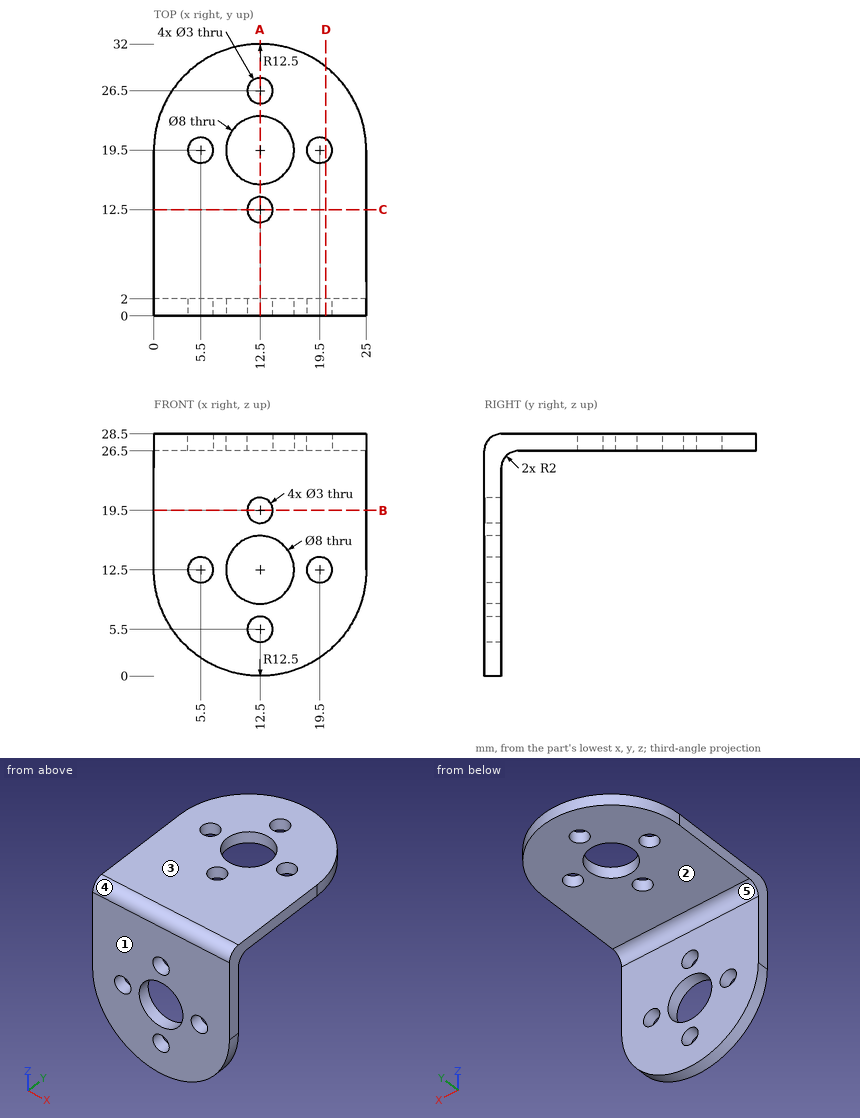
Could you check a few things on this drawing? It's one solid part, dimensions in mm from its lowest x, y, z. A direction names the side the tool comes from. Round coordinates to 2 decimals unless told otherwise and drop trailing zeros. Order: outer loops, then holes, each group sorted by start corner. A loop starts at its lowest first (then second) coordinate and runs counter-clockwise, first axis right, second up. Notation, with made-up numbers: M -4.75,59 L 18.25,59 A27 cw 18.25,95 Z; hole C 6,44.5 d9. An arc over 180 degrees is marked long. Return JSON: item names as keys, results as strings. Group by question number.
1. Please list where these lines run through material, in increasing order: probe 1 along Z at (x, y) = (6.25, 8); probe 2 along Y at (x, z) = (1.5, 23.75); probe 3 along Z at (x, y) = (5.5, 0.85).
2. I'm going to push flat-ended pins straight in: pin 1 Ø3 at (x, y) = (3.5, 8) entering from -Z; pin 2 Ø2.5 at (x, z) = (12.5, 19.5) entering from +Y; pin 3 Ø7.5 at (x, z) = (12, 9) entering from +Y. Where does each tip first touch, or does it pass through?
3. If we mould it in two halves opening along Y, with no side actions, what happens to the marked faces 3, 4 and 5? For each: pulls with the +Y half, pulls with the -Y half, needs draft (parallel to the pull), parting line crosses it, or undercut.
4. If we section it at A-A on x = 12.5: State how many separate pieces and enclosed holes the cut face has, then the cut area to 3 significant figures.
5. If we section it at C-C on y = 12.5: List the corners of the cut face in (x, z) for me.
6. If we section it at B-B on z = 19.5: List the corners of the cut face in (x, y) for me.
7. If we section it at D-D on x = 20.25: List the corners of the cut face in (y, z) for me, then the cut area to 3 significant figures.
8. On a 3-axis mill with a long thin cutter (end or side, diameter ignored), from which of +Z, -Z, +X, -X, +Y, -Y can I reach the whole of each face in a straight line? I mean the marked faces 1 and 2. Say none if no direction works.
Reply:
{
 "1": {"probe 1": "26.5 to 28.5", "probe 2": "0 to 2", "probe 3": "2.14 to 11, 14 to 28.14"},
 "2": {"pin 1": "z = 26.5", "pin 2": "through", "pin 3": "y = 2"},
 "3": {"face 3": "needs draft", "face 4": "pulls with the -Y half", "face 5": "pulls with the +Y half"},
 "4": {"separate pieces": "7", "enclosed holes": "0", "area": "61.0 mm^2"},
 "5": {"outline": "M 0,26.5 L 11,26.5 L 11,28.5 L 0,28.5 Z; M 14,26.5 L 25,26.5 L 25,28.5 L 14,28.5 Z"},
 "6": {"outline": "M 0,0 L 11,0 L 11,2 L 0,2 Z; M 14,0 L 25,0 L 25,2 L 14,2 Z"},
 "7": {"outline": "M 0,2.69 L 2,2.69 L 2,11.2 L 0,11.2 Z; M 0,13.8 L 2,13.8 L 2,24.5 A2 cw 4,26.5 L 18.2,26.5 L 18.2,28.5 L 2,28.5 A2 ccw 0,26.5 Z; M 20.8,26.5 L 29.31,26.5 L 29.31,28.5 L 20.8,28.5 Z", "area": "95.8 mm^2"},
 "8": {"face 1": "+Z, -Z, +X, -X, -Y", "face 2": "-Z, +X, -X, +Y"}
}
